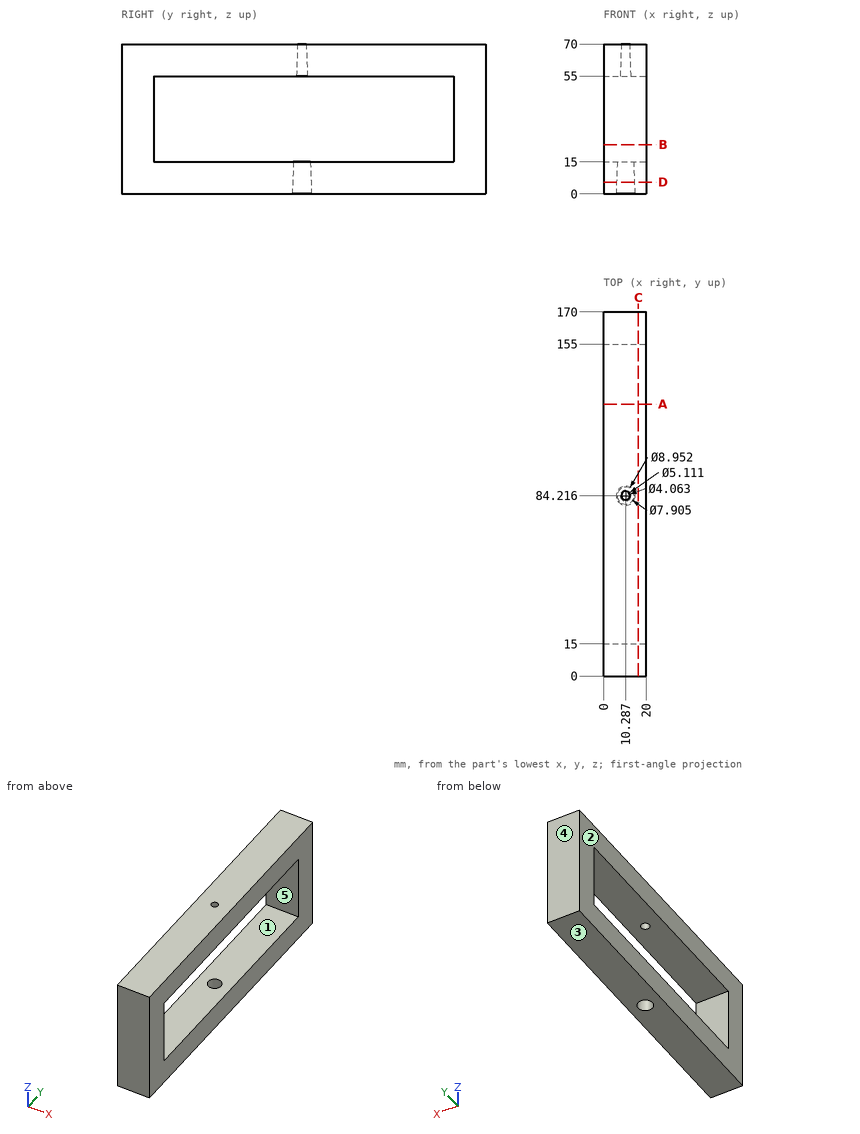
Answer from the drawing. Dimensions are ordinates in mm from the lowest x, y and z of the part. A direction names the side the tool comes from. Round coordinates to 2 decimals unless told otherwise and drop trailing zeros. Loops run counter-clockwise (first coordinate to the right, second up) from the corner with the lowest first, then second, coordinate; pieces in that order, holes last.
Q1. Section B-B on z = 23 is taken. Write down the section's boundary in (x, y), and give its area (3 significant figures).
Q2. Section C-C on x = 16.25 is taken. Write down the section's boundary in (y, z).
Q3. Section D-D on z = 5.5 is taken. Write down the section's boundary in (x, y) (1 decimal).
Q4. This flat-tipped pin is pushed along its axis until it touches: pin 1 (1.5 mm diameter, centred on y = 127, z = 52.5, fed in from -X). Where does it stop, or does it pass through?
Q5. Section A-A on y = 127 is taken. Write down the section's boundary in (x, z), and give its area (3 significant figures).
Q6. Which of the six approach directions +Z, -Z, +X, -X, +Y, -Y give full straight-line access (tool end or side, diameter ignored) to the marked faces 1 and 2?
Q7. Consider probe 1 along Z at (x, y) = (2.25, 86); probe 2 along Y at (x, z) = (11.25, 27); probe 3 along Y at (x, z) = (7.5, 7). Determine where each line is inside the solid, lowest interval first.
Q8. Determine the mould class of the marked faces 3, 4 and 5 for opening direction Z: released by +Z, released by -Z, zero draft, split by the parting line, or undercut.
Output:
1. outline: (0, 0) - (20, 0) - (20, 15) - (0, 15) - close; (0, 155) - (20, 155) - (20, 170) - (0, 170) - close
1. area: 600 mm2
2. outline: (0, 0) - (170, 0) - (170, 70) - (0, 70) - close; hole (15, 15) - (155, 15) - (155, 55) - (15, 55) - close
3. outline: (0, 0) - (20, 0) - (20, 170) - (0, 170) - close; hole circle Ø8.6 at (10.3, 84.2)
4. pin 1: passes through
5. outline: (0, 0) - (20, 0) - (20, 15) - (0, 15) - close; (0, 55) - (20, 55) - (20, 70) - (0, 70) - close
5. area: 600 mm2
6. face 1: +X, -X
6. face 2: +Z, -Z, -X, +Y, -Y
7. probe 1: z = 0 to 15, 55 to 70
7. probe 2: y = 0 to 15, 155 to 170
7. probe 3: y = 0 to 81.03, 87.4 to 170
8. face 3: released by -Z
8. face 4: zero draft
8. face 5: undercut
